Read the model definition and answer for the solid it produces. Units are mm, in the model's axes. A direction names the side the tool comes from. Give positions to 0.01 mm unless a question says otherwise; leave off trailing zeros. Order: outer loops, then holes, each group sorted by start corner. A loop starts at its lowest first (then second) coordinate and runs counter-clockwise, first axis right, second up. Notation, with made-up numbers: (10, 13) -> (17, 13) arc R20 ccw to (17, 21) -> close; hole circle Ø9 at (18, 4). An arc over 180 degrees is marked (long way). Use one line per item in the form item = value.
```python
from build123d import *

# Parameters (mm, degrees)
SKETCH1_W           = 32.5
SKETCH1_H           = 16
BOSS_EXTRUDE1_DEPTH = 1.5
SKETCH3_W           = 34.5
SKETCH3_H           = 18
SKETCH3_W_2         = 32.5
SKETCH3_H_2         = 16
BOSS_EXTRUDE2_DEPTH = 10.5
SKETCH4_W           = 5
SKETCH4_H           = 5
BOSS_EXTRUDE3_DEPTH = 2
SKETCH6_W           = 34.5
SKETCH6_H           = 5
BOSS_EXTRUDE5_DEPTH = 1.5
SKETCH7_R           = 1.5
CUT_EXTRUDE1_DEPTH  = 1.5
SKETCH8_W           = 2.5
SKETCH8_H           = 5
BOSS_EXTRUDE6_DEPTH = 9
SKETCH9_R           = 1.5
CUT_EXTRUDE2_DEPTH  = 37.47259245
SKETCH10_R          = 0.75
BOSS_EXTRUDE7_DEPTH = 2


with BuildPart() as part:
    # Sketch1 → Boss-Extrude1 (new body)
    with BuildSketch(Plane(origin=(0, 0, 0), x_dir=(1, 0, 0), z_dir=(0, 1, 0))):
        Rectangle(SKETCH1_W, SKETCH1_H)
    extrude(amount=BOSS_EXTRUDE1_DEPTH)

    # Sketch3 → Boss-Extrude2 (add)
    with BuildSketch(Plane(origin=(0, 0, 0), x_dir=(1, 0, 0), z_dir=(0, 1, 0))):
        Rectangle(SKETCH3_W, SKETCH3_H)
        Rectangle(SKETCH3_W_2, SKETCH3_H_2, mode=Mode.SUBTRACT)
    extrude(amount=BOSS_EXTRUDE2_DEPTH)

    # Sketch4 → Boss-Extrude3 (add)
    with BuildSketch(Plane(origin=(0, 1.5, 0), x_dir=(1, 0, 0), z_dir=(0, 1, 0))):
        with Locations((5.75, 5.5)):
            Rectangle(SKETCH4_W, SKETCH4_H)
        with Locations((5.75, -5.5)):
            Rectangle(SKETCH4_W, SKETCH4_H)
        with Locations((-8.75, 5.5)):
            Rectangle(SKETCH4_W, SKETCH4_H)
        with Locations((-8.75, -5.5)):
            Rectangle(SKETCH4_W, SKETCH4_H)
    extrude(amount=BOSS_EXTRUDE3_DEPTH)

    # Sketch6 → Boss-Extrude5 (add)
    with BuildSketch(Plane(origin=(0, 0, 0), x_dir=(1, 0, 0), z_dir=(0, 1, 0))):
        with Locations((0, 11.5)):
            Rectangle(SKETCH6_W, SKETCH6_H)
        with Locations((0, -11.5)):
            Rectangle(SKETCH6_W, SKETCH6_H)
    extrude(amount=BOSS_EXTRUDE5_DEPTH)

    # Sketch7 → Cut-Extrude1 (cut)
    with BuildSketch(Plane(origin=(0, 1.5, 0), x_dir=(1, 0, 0), z_dir=(0, 1, 0))):
        with Locations(Location((5.25, 12, 0), (0, 0, 270))):
            Circle(SKETCH7_R)
        with Locations(Location((5.25, -12, 0), (0, 0, 90))):
            Circle(SKETCH7_R)
    extrude(amount=-CUT_EXTRUDE1_DEPTH, mode=Mode.SUBTRACT)

    # Sketch8 → Boss-Extrude6 (add)
    with BuildSketch(Plane(origin=(0, 1.5, 0), x_dir=(1, 0, 0), z_dir=(0, 1, 0))):
        with Locations((-16, 11.5)):
            Rectangle(SKETCH8_W, SKETCH8_H)
        with Locations((-16, -11.5)):
            Rectangle(SKETCH8_W, SKETCH8_H)
    extrude(amount=BOSS_EXTRUDE6_DEPTH)

    # Sketch9 → Cut-Extrude2 (cut, through all)
    with BuildSketch(Plane(origin=(-14.75, 0, 0), x_dir=(0, 0, -1), z_dir=(1, 0, 0))):
        with Locations((12, 5)):
            Circle(SKETCH9_R)
        with Locations(Location((-12, 5, 0), (0, 0, 180))):
            Circle(SKETCH9_R)
    extrude(amount=-CUT_EXTRUDE2_DEPTH, mode=Mode.SUBTRACT)

    # Sketch10 → Boss-Extrude7 (add)
    with BuildSketch(Plane(origin=(0, 3.5, 0), x_dir=(1, 0, 0), z_dir=(0, 1, 0))):
        with Locations(Location((6.25, 5, 0), (0, 0, 90))):
            Circle(SKETCH10_R)
        with Locations(Location((6.25, -5, 0), (0, 0, 90))):
            Circle(SKETCH10_R)
    extrude(amount=BOSS_EXTRUDE7_DEPTH)


solid = part.part
```
Item 1: The part is cut by section D-D on x = -4. Give the vertices of the cut face in (y, z), and give its area (3 significant figures).
Checks:
outline = (0, -14) -> (1.5, -14) -> (1.5, -9) -> (10.5, -9) -> (10.5, -8) -> (1.5, -8) -> (1.5, 8) -> (10.5, 8) -> (10.5, 9) -> (1.5, 9) -> (1.5, 14) -> (0, 14) -> close
area = 60.0 mm²
Item 2: The part is cut by section B-B on z = -5. Give the vertices of the cut face in (x, y), and give its area (4 significant figures).
Checks:
outline = (-17.25, 0) -> (17.25, 0) -> (17.25, 10.5) -> (16.25, 10.5) -> (16.25, 1.5) -> (8.25, 1.5) -> (8.25, 3.5) -> (7, 3.5) -> (7, 5.5) -> (5.5, 5.5) -> (5.5, 3.5) -> (3.25, 3.5) -> (3.25, 1.5) -> (-6.25, 1.5) -> (-6.25, 3.5) -> (-11.25, 3.5) -> (-11.25, 1.5) -> (-16.25, 1.5) -> (-16.25, 10.5) -> (-17.25, 10.5) -> close
area = 92.75 mm²
Item 3: The part is cut by section C-C on y = 8.5. Give the vertices of the cut face in (x, z), and give its area (3 significant figures).
Checks:
outline = (-17.25, -14) -> (-14.75, -14) -> (-14.75, -9) -> (17.25, -9) -> (17.25, 9) -> (-14.75, 9) -> (-14.75, 14) -> (-17.25, 14) -> close; hole (-16.25, -8) -> (16.25, -8) -> (16.25, 8) -> (-16.25, 8) -> close
area = 126 mm²
Item 4: Determine the mould class of faces 1 (the flat face through (6, 2, -3)), 2 (the flat face through (-5, 1, 14)), 3 (the flat face through (-14.75, 7, -11)) for opening direction Z: +Z half, -Z half, draft (parallel to the pull), parting line (faces both ways), or undercut.
Checks:
face_1 = undercut
face_2 = +Z half
face_3 = draft
Item 5: The part is cut by section A-A on y = 5. Give the vertices of the cut face in (x, z).
Checks:
outline = (-17.25, -14) -> (-14.75, -14) -> (-14.75, -13.5) -> (-17.25, -13.5) -> close; (-17.25, -10.5) -> (-14.75, -10.5) -> (-14.75, -9) -> (17.25, -9) -> (17.25, 9) -> (-14.75, 9) -> (-14.75, 10.5) -> (-17.25, 10.5) -> close; (-17.25, 13.5) -> (-14.75, 13.5) -> (-14.75, 14) -> (-17.25, 14) -> close; circle Ø1.5 at (6.25, -5); circle Ø1.5 at (6.25, 5); hole (-16.25, -8) -> (16.25, -8) -> (16.25, 8) -> (-16.25, 8) -> close
Item 6: Given pin 1 Ø4.5 at (x, y) = (-0.5, 4.5) entering from +Z; pin 2 Ø5 at (x, z) = (-2.5, -3) entering from +Y; pin 3 Ø2.5 at (x, z) = (5.25, 12) entering from +Y; pin 4 Ø2.5 at (x, y) = (-4.5, 5) entering from -Z, each flat-ended and moving along its own axis, determine where each tip first touches the part or whether it passes through.
Checks:
pin_1 = 9
pin_2 = 1.5
pin_3 = through
pin_4 = -9
Item 7: Straight lines are drawn through the part: L1, parallel to X at y = 2.25, z = 4.5; L2, parallel to Z at x = -11.5, y = 7; L3, parallel to X at y = 4.5, z = -5.5. For each, find the intervals that lie inside material, in ascending order. Write a range as from..to.
Checks:
L1 = -17.25..-16.25, -11.25..-6.25, 3.25..8.25, 16.25..17.25
L2 = -9..-8, 8..9
L3 = -17.25..-16.25, 5.69..6.81, 16.25..17.25
Item 8: Which of the six approach directions +Z, -Z, +X, -X, +Y, -Y give full straight-line access (tool end or side, diameter ignored) to faces 4 (the flat face through (-5, 1, -14)), 5 (the flat face through (-9, 3.5, -6))?
Checks:
face_4 = -Z, +X, -X, +Y, -Y
face_5 = +Y
